Geometry: see drawing. Coordinates: mm, zero at the bounding-box minimum. A direction names the side the tool comes from. Coordinates: 2 decimals unless noted, no trailing zeros. Order: outer loops, then holes, each group sorted by start corner. A loop starts at its lowest first (then second) coordinate and runs counter-clockwise, first axis right, second up. Notation, with made-up numbers: (-24, 19.5) -> (26, 19.5) arc R13 cw to (26, 23.5) -> close; hole circle Ø3 at (85.5, 72.25). An arc over 180 degrees is marked (long way). One line per item, written item: value. Start each with the question number.
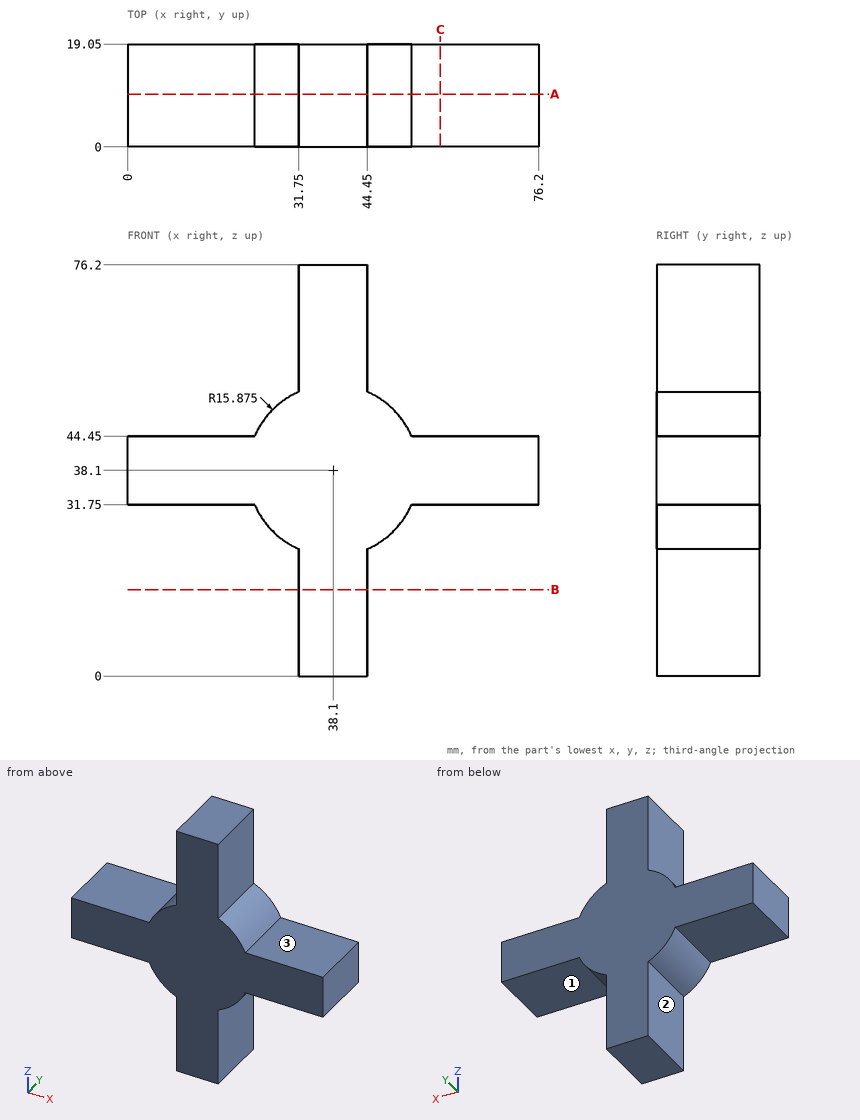
1) Section query A-A, the plane y = 9.75. Return the cut outline in (x, z) (3 decimals).
2) Pin query (flat end, axial travel): pin 1 Ø6 at (y, z) = (12.5, 31.5) entering from +X; pin 2 Ø5 at (y, z) = (5, 11) entering from -X; pin 3 Ø8 at (y, z) = (14, 26) entering from +X; pin 4 Ø1.5 at (x, y) = (19.5, 16) entering from +Z. Return the tip coordinate at first contact, or that it passes through.
3) Ray query, line 1 along X through (y, z) = (17.5, 53.5); line 2 along X through (y, z) = (2.5, 25). Return the intervals inside material, ascending. Write a range as from..to.
4) Section query C-C, the plane x = 58. Return the cut outline in (y, z).
5) Access query for the marked faces 1, 2 and 3. Directions: +Z, -Z, +X, -X, +Y, -Y. A direction counts if a zero-diameter tool reaches every point of the face in a straight line with its end or side. Return the directions, or none.
6) Section query B-B, the plane z = 16. Return the cut outline in (x, y).
Entries:
1. outline: (0, 31.75) -> (23.55, 31.75) arc R15.875 ccw to (31.75, 23.55) -> (31.75, 0) -> (44.45, 0) -> (44.45, 23.55) arc R15.875 ccw to (52.65, 31.75) -> (76.2, 31.75) -> (76.2, 44.45) -> (52.65, 44.45) arc R15.875 ccw to (44.45, 52.65) -> (44.45, 76.2) -> (31.75, 76.2) -> (31.75, 52.65) arc R15.875 ccw to (23.55, 44.45) -> (0, 44.45) -> close
2. pin 1: stops at x = 76.2
2. pin 2: stops at x = 31.75
2. pin 3: stops at x = 51.75
2. pin 4: stops at z = 44.45
3. line 1: x = 31.75..44.45
3. line 2: x = 29.13..47.07
4. outline: (0, 31.75) -> (19.05, 31.75) -> (19.05, 44.45) -> (0, 44.45) -> close
5. face 1: -Z, +X, +Y, -Y
5. face 2: -Z, -X, +Y, -Y
5. face 3: +Z, +X, +Y, -Y
6. outline: (31.75, 0) -> (44.45, 0) -> (44.45, 19.05) -> (31.75, 19.05) -> close
